Model file for the job. Use its own axes, mm. A direction names the side the tool comes from. Coordinates: 2 decimals unless noted, no trailing zeros. Order: outer loops, then holes, each group sorted by start corner. A loop starts at its lowest first (then second) coordinate and runs counter-clockwise, first axis right, second up. Notation, with made-up numbers: M 31,64.5 L 44,64.5 A11 ccw 44,80.5 Z; hole C -32,81.25 d3. An arc over 180 degrees is marked long. Return JSON: item names as keys, results as strings.
```python
from build123d import *

# Parameters (mm, degrees)
FUNNEL_RIGHT_SIDE_DEPTH = 170
FILLET2_R               = 10
FILLET3_R               = 2.5


with BuildPart() as part:
    # Sketch1 → Funnel - Right Side (new body)
    with BuildSketch(Plane.XY):
        Polygon((0, 0), (0, 97.1), (41.974030913, 147.122702136), (36.974030913, 147.122702136), (-30, 67.306160185), (-5, 36.081170193), (-5, 0), align=None)
    extrude(amount=FUNNEL_RIGHT_SIDE_DEPTH)

    # Fillet2
    fillet2_edges = [part.edges().sort_by_distance(p)[0] for p in [
        (-5, 36.081170193, 85),
        (0, 97.1, 85),
    ]]
    fillet(fillet2_edges, radius=FILLET2_R)

    # Fillet3
    fillet3_edges = [part.edges().sort_by_distance(p)[0] for p in [
        (-30, 67.306160185, 85),
    ]]
    fillet(fillet3_edges, radius=FILLET3_R)


solid = part.part
```
Item 1: Pull direction Z, two halves, no side cores. Call faces 1 (the flat face through (-7, 68, 170)), 2 (the flat face through (-7, 68, 0)), 3 (the cylindrical face through (-5.58, 35.93, 86.19)): +Z half, -Z half, draft (parallel to the pull), parting line (faces both ways), or undercut.
Check result:
{"face 1": "+Z half", "face 2": "-Z half", "face 3": "draft"}
Item 2: Saw through at B-B (y = 108). Write the cut outline in (x, z), and give its area (3 significant figures).
Check result:
{"outline": "M 4.15,0 L 9.15,0 L 9.15,170 L 4.15,170 Z", "area": "850 mm2"}
Item 3: Wall check: line 1 (X direction, y = 16.5, z = 12.5); line 2 (X direction, y = 66.5, z = 77.5); line 3 (Y direction, x = -25.5, z = 53.5). Give the ranges that are in metal, low to high.
Check result:
{"line 1": "x = -5 to 0", "line 2": "x = -29.15 to 0", "line 3": "y = 61.69 to 72.67"}
Item 4: Saw through at A-A (z = 45). Write the cut outline in (x, y), and give its area (3 significant figures).
Check result:
{"outline": "M -28.72,65.71 L -7.19,38.82 A10 cw -5,32.57 L -5,0 L 0,0 L 0,93.46 A10 cw 2.34,99.89 L 41.97,147.12 L 36.97,147.12 L -28.68,68.88 A2.5 ccw Z", "area": "1,500 mm2"}
Item 5: Drop flat-ended pins along their axis: pin 1 Ø4 at (y, z) = (89.5, 142) entering from -X; pin 2 Ø6 at (y, z) = (31.5, 136) entering from -X; pin 3 Ø10 at (y, z) = (51, 42) entering from -X. Give the stop position or say it passes through.
Check result:
{"pin 1": "stops at x = -13.06", "pin 2": "stops at x = -5.19", "pin 3": "stops at x = -20.95"}
Item 6: 3-axis set-ups, long thin cutter, end or side, ignore diameter. For faces 4 (the flat face through (-5, 17, 84)), 5 (the flat face through (0, 46, 84)), 6 (the flat face through (-3, 0, 84)): which of +Z, -Z, +X, -X, +Y, -Y reach the whole face in a straight line?
Check result:
{"face 4": "+Z, -Z, -X, -Y", "face 5": "+Z, -Z, +X, -Y", "face 6": "+Z, -Z, +X, -X, -Y"}
Item 7: Saw through at C-C (x = -18). Write the cut outline in (y, z).
Check result:
{"outline": "M 52.32,0 L 81.61,0 L 81.61,170 L 52.32,170 Z"}
